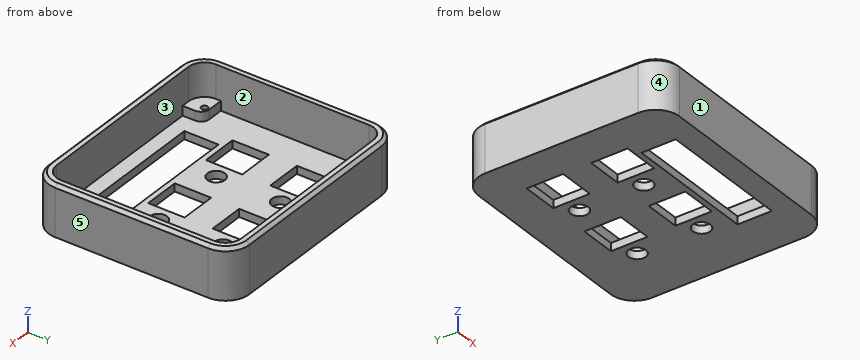
from build123d import *

# Parameters (mm, degrees)
F0_R     = 1
F1_DEPTH = 16
F2_T     = -2.5
F3_DEPTH = 5.5
F4_W     = 41.64
F4_H     = 10.8
F4_R     = 2.75
F4_W_2   = 11.5
F4_H_2   = 11.5
F5_DEPTH = 2.501
F6_SIZE  = 1


with BuildPart() as f1:
    # F0 (on Top) → F1 (new body)
    with BuildSketch(Plane.XY):
        with BuildLine():
            ThreePointArc((36.115, 24.13), (33.906585, 29.461585), (28.575, 31.67))
            Line((28.575, 31.67), (26.035, 31.67))
            Line((26.035, 31.67), (26.035, 25.185541))
            ThreePointArc((26.035, 25.185541), (26.778949, 23.38949), (28.575, 22.645541))
            Line((28.575, 22.645541), (36.115, 22.645541))
            Line((36.115, 22.645541), (36.115, 24.13))
        make_face()
        with Locations((28.575, 24.13)):
            Circle(F0_R, mode=Mode.SUBTRACT)
        with BuildLine():
            Line((-26.035, 25.185541), (-26.035, 31.67))
            Line((-26.035, 31.67), (-28.575, 31.67))
            ThreePointArc((-28.575, 31.67), (-33.906585, 29.461585), (-36.115, 24.13))
            Line((-36.115, 24.13), (-36.115, 22.645541))
            Line((-36.115, 22.645541), (-28.575, 22.645541))
            ThreePointArc((-28.575, 22.645541), (-26.778949, 23.38949), (-26.035, 25.185541))
        make_face()
        with Locations((-28.575, 24.13)):
            Circle(F0_R, mode=Mode.SUBTRACT)
        with BuildLine():
            Line((36.115, -24.13), (36.115, -22.645541))
            Line((36.115, -22.645541), (28.575, -22.645541))
            ThreePointArc((28.575, -22.645541), (26.778949, -23.38949), (26.035, -25.185541))
            Line((26.035, -25.185541), (26.035, -31.67))
            Line((26.035, -31.67), (28.575, -31.67))
            ThreePointArc((28.575, -31.67), (33.906585, -29.461585), (36.115, -24.13))
        make_face()
        with Locations((28.575, -24.13)):
            Circle(F0_R, mode=Mode.SUBTRACT)
        with BuildLine():
            Line((-28.575, -22.645541), (-36.115, -22.645541))
            Line((-36.115, -22.645541), (-36.115, -24.13))
            ThreePointArc((-36.115, -24.13), (-33.906585, -29.461585), (-28.575, -31.67))
            Line((-28.575, -31.67), (-26.035, -31.67))
            Line((-26.035, -31.67), (-26.035, -25.185541))
            ThreePointArc((-26.035, -25.185541), (-26.778949, -23.38949), (-28.575, -22.645541))
        make_face()
        with Locations((-28.575, -24.13)):
            Circle(F0_R, mode=Mode.SUBTRACT)
        with BuildLine():
            Line((26.035, 25.185541), (26.035, 31.67))
            Line((26.035, 31.67), (-26.035, 31.67))
            Line((-26.035, 31.67), (-26.035, 25.185541))
            ThreePointArc((-26.035, 25.185541), (-26.778949, 23.38949), (-28.575, 22.645541))
            Line((-28.575, 22.645541), (-36.115, 22.645541))
            Line((-36.115, 22.645541), (-36.115, -22.645541))
            Line((-36.115, -22.645541), (-28.575, -22.645541))
            ThreePointArc((-28.575, -22.645541), (-26.778949, -23.38949), (-26.035, -25.185541))
            Line((-26.035, -25.185541), (-26.035, -31.67))
            Line((-26.035, -31.67), (26.035, -31.67))
            Line((26.035, -31.67), (26.035, -25.185541))
            ThreePointArc((26.035, -25.185541), (26.778949, -23.38949), (28.575, -22.645541))
            Line((28.575, -22.645541), (36.115, -22.645541))
            Line((36.115, -22.645541), (36.115, 22.645541))
            Line((36.115, 22.645541), (28.575, 22.645541))
            ThreePointArc((28.575, 22.645541), (26.778949, 23.38949), (26.035, 25.185541))
        make_face()
        with Locations((-28.575, 24.13)):
            Circle(F0_R)
        with Locations((28.575, 24.13)):
            Circle(F0_R)
        with Locations((28.575, -24.13)):
            Circle(F0_R)
        with Locations((-28.575, -24.13)):
            Circle(F0_R)
    extrude(amount=F1_DEPTH)

    # F2
    f2_openings = [f1.faces().sort_by_distance(p)[0] for p in [
        (0, 0, 16),
    ]]
    offset(amount=F2_T, openings=f2_openings)

    # F0 (on Top) → F3 (join)
    with BuildSketch(Plane.XY):
        with BuildLine():
            Line((-28.575, -22.645541), (-36.115, -22.645541))
            Line((-36.115, -22.645541), (-36.115, -24.13))
            ThreePointArc((-36.115, -24.13), (-33.906585, -29.461585), (-28.575, -31.67))
            Line((-28.575, -31.67), (-26.035, -31.67))
            Line((-26.035, -31.67), (-26.035, -25.185541))
            ThreePointArc((-26.035, -25.185541), (-26.778949, -23.38949), (-28.575, -22.645541))
        make_face()
        with Locations((-28.575, -24.13)):
            Circle(F0_R, mode=Mode.SUBTRACT)
        with BuildLine():
            Line((36.115, -24.13), (36.115, -22.645541))
            Line((36.115, -22.645541), (28.575, -22.645541))
            ThreePointArc((28.575, -22.645541), (26.778949, -23.38949), (26.035, -25.185541))
            Line((26.035, -25.185541), (26.035, -31.67))
            Line((26.035, -31.67), (28.575, -31.67))
            ThreePointArc((28.575, -31.67), (33.906585, -29.461585), (36.115, -24.13))
        make_face()
        with Locations((28.575, -24.13)):
            Circle(F0_R, mode=Mode.SUBTRACT)
        with BuildLine():
            ThreePointArc((36.115, 24.13), (33.906585, 29.461585), (28.575, 31.67))
            Line((28.575, 31.67), (26.035, 31.67))
            Line((26.035, 31.67), (26.035, 25.185541))
            ThreePointArc((26.035, 25.185541), (26.778949, 23.38949), (28.575, 22.645541))
            Line((28.575, 22.645541), (36.115, 22.645541))
            Line((36.115, 22.645541), (36.115, 24.13))
        make_face()
        with Locations((28.575, 24.13)):
            Circle(F0_R, mode=Mode.SUBTRACT)
        with BuildLine():
            Line((-26.035, 25.185541), (-26.035, 31.67))
            Line((-26.035, 31.67), (-28.575, 31.67))
            ThreePointArc((-28.575, 31.67), (-33.906585, 29.461585), (-36.115, 24.13))
            Line((-36.115, 24.13), (-36.115, 22.645541))
            Line((-36.115, 22.645541), (-28.575, 22.645541))
            ThreePointArc((-28.575, 22.645541), (-26.778949, 23.38949), (-26.035, 25.185541))
        make_face()
        with Locations((-28.575, 24.13)):
            Circle(F0_R, mode=Mode.SUBTRACT)
    extrude(amount=F3_DEPTH)

    # F4 (on face) → F5 (cut, through all)
    with BuildSketch(Plane.XY.offset(2.5)):
        with Locations((0.365, -19.16)):
            Rectangle(F4_W, F4_H)
        with Locations((17.088419, -5.397456)):
            Circle(F4_R)
        with Locations((6.585, 13.97)):
            Rectangle(F4_W_2, F4_H_2)
        with Locations((17.088419, 14.922544)):
            Circle(F4_R)
        with Locations((6.585, -6.35)):
            Rectangle(F4_W_2, F4_H_2)
        with Locations((-18.415, -6.35)):
            Rectangle(F4_W_2, F4_H_2)
        with Locations((-7.911581, -5.397456)):
            Circle(F4_R)
        with Locations((-18.415, 13.97)):
            Rectangle(F4_W_2, F4_H_2)
        with Locations((-7.911581, 14.922544)):
            Circle(F4_R)
    extrude(amount=-F5_DEPTH, mode=Mode.SUBTRACT)

    # F6
    f6_edges = [f1.edges().sort_by_distance(p)[0] for p in [
        (36.115, 0, 16),
    ]]
    chamfer(f6_edges, length=F6_SIZE)


solid = f1.part
Source: CAD feature listing. Evaluate the final solid. Frame: model axes, mm. Face numbers are marked on the shaded views. A direction names the side the tool comes from. Give positions to 0.01 mm unless a question says otherwise; leave off trailing zeros. Write each loop counter-clockwise with the first axis right and the second up, starting at its lowest first coordinate (ties: lowest second). Pieces come first, ordered by that corner, then holes. Notation, with made-up numbers: M 66,6.25 L 73,6.25 A27 cw 73,40.25 Z; hole C -6,-37.75 d3. An arc over 180 degrees is marked long. Return JSON: item names as keys, results as strings. Group by question number.
1) Cut plane B-B, the plane x = 10. Output: boundary loops of the cut face in (y, z).
2) Cut plane C-C, the plane z = 9.75. Output: boundary loops of the cut face in (x, y) (3 decimals).
3) Ray query, L1, parallel to X at y = 10.5, z = 1 (3 decimals); L2, parallel to Y at x = -20.5, z = 15; L3, parallel to X at y = -12, z = 13 (3 decimals). Return the intervals inside material, ascending.
4) Draft query along X for the marked faces 3, 4 and 5. Return one class per face: released by +X, released by -X, zero draft, split by the parting line, or undercut.
5) First-contact query: pin 1 Ø0.9 at (y, z) = (-26.5, 4.5) entering from -X; pin 2 Ø8 at (x, y) = (-7, -4.5) entering from +Z; pin 3 Ø7 at (x, y) = (29, -24.5) entering from +Z. Flat tips, straight axial feed; report the tip coordinate or a pass-through.
6) Cut plane A-A, the plane y = -9.5. Output: boundary loops of the cut face in (x, z) (3 decimals).
7) Cut plane D-D, the plane y = 4.5. Output: boundary loops of the cut face in (x, z) (3 decimals).
8) Set-up query: the marked faces 1 and 2. Return all of +Z, -Z, +X, -X, +Y, -Y with unobstructed straight access to the full face (end or side cutting, diameter ignored); none if empty.
Data:
{
 "1": {"outline": "M -31.67,0 L -24.56,0 L -24.56,2.5 L -29.17,2.5 L -29.17,16 L -30.67,16 L -31.67,15 Z; M -13.76,0 L -12.1,0 L -12.1,2.5 L -13.76,2.5 Z; M -0.6,0 L 8.22,0 L 8.22,2.5 L -0.6,2.5 Z; M 19.72,0 L 31.67,0 L 31.67,15 L 30.67,16 L 29.17,16 L 29.17,2.5 L 19.72,2.5 Z"},
 "2": {"outline": "M -36.115,-24.13 A7.54 ccw -28.575,-31.67 L 28.575,-31.67 A7.54 ccw 36.115,-24.13 L 36.115,24.13 A7.54 ccw 28.575,31.67 L -28.575,31.67 A7.54 ccw -36.115,24.13 Z; hole M -33.615,-24.13 A5.04 ccw -28.575,-29.17 L 28.575,-29.17 A5.04 ccw 33.615,-24.13 L 33.615,24.13 A5.04 ccw 28.575,29.17 L -28.575,29.17 A5.04 ccw -33.615,24.13 Z"},
 "3": {"L1": "x = -36.115 to -24.165, -12.665 to 0.835, 12.335 to 36.115", "L2": "y = -31.67 to -29.17, 29.17 to 31.67", "L3": "x = -36.115 to -33.615, 33.615 to 36.115"},
 "4": {"face 3": "undercut", "face 4": "released by -X", "face 5": "released by +X"},
 "5": {"pin 1": "stops at x = -35.87", "pin 2": "stops at z = 2.5", "pin 3": "stops at z = 5.5"},
 "6": {"outline": "M -36.115,0 L -24.165,0 L -24.165,2.5 L -33.615,2.5 L -33.615,16 L -35.115,16 L -36.115,15 Z; M -12.665,0 L 0.835,0 L 0.835,2.5 L -12.665,2.5 Z; M 12.335,0 L 36.115,0 L 36.115,15 L 35.115,16 L 33.615,16 L 33.615,2.5 L 12.335,2.5 Z"},
 "7": {"outline": "M -36.115,0 L 36.115,0 L 36.115,15 L 35.115,16 L 33.615,16 L 33.615,2.5 L -33.615,2.5 L -33.615,16 L -35.115,16 L -36.115,15 Z"},
 "8": {"face 1": "+Z, -Z, +X, -X, -Y", "face 2": "+Z"}
}
